Read the model definition and answer for the solid it produces. Units are mm, in the model's axes. A direction names the side the tool comes from. Give positions to 0.01 mm unless a question says otherwise; leave off trailing zeros. Order: outer loops, then holes, each group sorted by start corner. A loop starts at its lowest first (then second) coordinate and runs counter-clockwise, first axis right, second up. Notation, with made-up numbers: (15, 36) - (74, 36) arc R23 ccw to (74, 49) - close; hole circle Ø7 at (79.25, 89.5). An arc over 180 degrees is marked (long way). Write item = value, one per line.
```python
from build123d import *

# Parameters (mm, degrees)
F0_R     = 16.51
F1_DEPTH = 44.45
F2_R     = 2.286
F3_DEPTH = 27.178
F4_W     = 10.16
F4_H     = 2.54
F5_DEPTH = 7.62


with BuildPart() as f1:
    # F0 (on Front) → F1 (new body)
    with BuildSketch(Plane.XZ):
        Circle(F0_R)
    extrude(amount=F1_DEPTH)

    # F2 (on face) → F3 (join)
    with BuildSketch(Plane.XZ.offset(44.45)):
        Circle(F2_R)
    extrude(amount=F3_DEPTH)

    # F4 (on face) → F5 (join)
    with BuildSketch(Plane(origin=(0, 0, 0), x_dir=(-1, 0, 0), z_dir=(0, 1, 0))):
        with Locations((-8.658255, 1.27)):
            Rectangle(F4_W, F4_H)
        with Locations((7.64519, 1.27)):
            Rectangle(F4_W, F4_H)
    extrude(amount=F5_DEPTH)


solid = f1.part
```
1. Section B-B (y = -42.5) is taken. Determine the outline of the cut face in (x, z), and give its area (3 significant figures).
Recorded:
outline = circle Ø33.02 at (0, 0)
area = 856 mm^2
2. Determine the mould class of faces 1 (the face through (13.738, 4, 1)), 2 (the face through (9, 4, 2.54)), 3 (the face through (3.578, 4, 1)) for opening direction X: +X half, -X half, draft (parallel to the pull), parting line (faces both ways), or undercut.
Recorded:
face_1 = +X half
face_2 = draft
face_3 = undercut
3. Section A-A (x = 0) is taken. Determine the outline of the cut face in (y, z).
Recorded:
outline = (-71.63, -2.29) - (-44.45, -2.29) - (-44.45, -16.51) - (0, -16.51) - (0, 16.51) - (-44.45, 16.51) - (-44.45, 2.29) - (-71.63, 2.29) - close
4. Flat-ended cylindrical pins translate along their axes: pin 1 (5 mm diameter, centred on y = -39.5, z = 7.5, fed in from -X); pin 2 (1.3 mm diameter, centred on y = 5.5, z = 2, fed in from -X); pin 3 (4 mm diameter, centred on x = 10, y = 4.5, fed in from +Z); pin 4 (10 mm diameter, centred on x = 7.5, y = -62, fed in from +Z). Find the tip coordinate at first contact, or state that the pin passes through.
Recorded:
pin_1 = -15.73
pin_2 = -12.73
pin_3 = 2.54
pin_4 = through
5. For faces 4 (the face through (-0.5, -57.85, -2.23)), 5 (the face through (-8, 4, 0)), 6 (the face through (-8, 4, 2.54)), 7 (the face through (-12.725, 4, 1)), determine the directions among +Z, -Z, +X, -X, +Y, -Y from which every point of the face is accessible in a straight line to the end or side of a thin tool.
Recorded:
face_4 = -Y
face_5 = -Z, +X, -X, +Y
face_6 = +Z, +X, -X, +Y
face_7 = +Z, -Z, -X, +Y
6. Straight lines are drawn through the part: L1, parallel to Y at x = -3.5, z = -1.5; L2, parallel to Z at x = 0, y = -51; L3, parallel to Y at x = -7.5, z = 2. For each, find the intervals that lie inside material, in ascending order. Write a range as [from, to].
Recorded:
L1 = [-44.45, 0]
L2 = [-2.29, 2.29]
L3 = [-44.45, 7.62]
7. Section D-D (x = -9.5) is taken. Determine the outline of the cut face in (y, z), and give its area (3 significant figures).
Recorded:
outline = (-44.45, -13.5) - (0, -13.5) - (0, 0) - (7.62, 0) - (7.62, 2.54) - (0, 2.54) - (0, 13.5) - (-44.45, 13.5) - close
area = 1,220 mm^2
8. Section C-C (z = 8.5) is taken. Determine the outline of the cut face in (x, y).
Recorded:
outline = (-14.15, -44.45) - (14.15, -44.45) - (14.15, 0) - (-14.15, 0) - close
